Autodesk Inventor part; units mm, degrees
ref_plane "YZ Plane" through (0, 0, 0) normal (1, 0, 0) x (0, 1, 0)
ref_plane "XZ Plane" through (0, 0, 0) normal (0, 1, 0) x (-1, 0, 0)
ref_plane "XY Plane" through (0, 0, 0) normal (0, 0, 1) x (1, 0, 0)
sketch "Panel" plane through (0, 0, 0) normal (0, 0, 1) x (1, 0, 0)
  line L0 (-190.5, 127) -> (190.5, 127)
  line L1 (190.5, 127) -> (190.5, -127)
  line L2 (190.5, -127) -> (-190.5, -127)
  line L3 (-190.5, -127) -> (-190.5, 127)
  point P0 (0, 0)
  point P1 (-190.5, 0)
  point P2 (0, 127)
  dimension "d0" = 254
  dimension "d3" = 381
sketch "JoystickMount" plane through (0, 0, 0) normal (0, 0, 1) x (1, 0, 0)
  line L0 (-114.625, 55.25) -> (-114.625, 14.75) construction
  line L1 (-114.625, 14.75) -> (-29.625, 14.75) construction
  point P0 (0, 0)
  point P1 (-72.125, 35)
  point P2 (-29.625, 55.25)
  point P3 (-114.625, 35)
  point P4 (-72.125, 14.75)
  dimension "d4" = 40.5
  dimension "d6" = 85
  dimension "d19" = 35
  dimension "d45" = 72.125
sketch "ButtonMounts" plane through (0, 0, 0) normal (0, 0, 1) x (1, 0, 0)
  line L0 (54.125, 74) -> (54.125, 35) construction
  line L1 (54.125, 35) -> (90.125, 35) construction
  point P0 (0, 0)
  point P1 (22.875, 56)
  point P2 (22.875, 17)
  point P3 (90.125, 74)
  point P4 (125.125, 65)
  point P5 (125.125, 26)
  point P6 (-72.125, 35)
  point P7 (72.125, 54.5)
  point P8 (54.125, 54.5)
  point P9 (72.125, 35)
  dimension "d7" = 39
  dimension "d9" = 39
  dimension "d10" = 39
  dimension "d11" = 39
  dimension "d12" = 31.25
  dimension "d13" = 36
  dimension "d14" = 35
  dimension "d15" = 18
  dimension "d16" = 9
  dimension "d55" = 144.25
  dimension "d56" = 72.125
extrude "PanelExtrusion" add sketch "Panel" against normal blind 3.175
hole "JoystickScrews" at (-29.625, 14.75, 0) at (-29.625, 55.25, 0) at (-114.625, 55.25, 0) at (-114.625, 14.75, 0) direction (0, 0, -1) diameter 4.5 end through all countersink diameter 9.4 countersink angle 90
hole "JoystickShaft" at (-72.125, 35, 0) direction (0, 0, -1) diameter 24 end through all
hole "ButtonHoles" at (125.125, 26, 0) at (90.125, 35, 0) at (90.125, 74, 0) at (125.125, 65, 0) at (54.125, 74, 0) at (54.125, 35, 0) at (22.875, 56, 0) at (22.875, 17, 0) direction (0, 0, -1) diameter 30 end through all
fillet "Corners" radius 1 4 edges at (190.5, 127, -1.5875) (190.5, -127, -1.5875) (-190.5, 127, -1.5875) (-190.5, -127, -1.5875)
ref_plane "10DegOffsetAlignment" through (190.5, -127, -3.175) normal (0, -0.9848, 0.1736) x (-1, 0, 0)
sketch "ScrewHoleCenters" plane through (0, 0, 0) normal (0, 0, 1) x (1, 0, 0)
  line L0 (-190.5, -126) -> (-190.5, 126)
  line L1 (-177.8, 89.411) -> (-180.975, 89.411)
  line L2 (-180.975, 85.6137) -> (-177.8, 85.6137)
  line L3 (-177.8, -85.9663) -> (-180.975, -85.9663)
  line L4 (-180.975, -89.7636) -> (-177.8, -89.7636)
  line L5 (177.8, -89.7636) -> (180.975, -89.7636)
  line L6 (180.975, -85.9663) -> (177.8, -85.9663)
  line L7 (177.8, 85.6137) -> (180.975, 85.6137)
  line L8 (180.975, 89.411) -> (177.8, 89.411)
  line L9 (-180.975, 89.411) -> (-180.975, 85.6137) construction
  line L10 (-177.8, 85.6137) -> (-177.8, 89.411) construction
  line L11 (-180.975, -85.9663) -> (-180.975, -89.7636) construction
  line L12 (-177.8, -89.7636) -> (-177.8, -85.9663) construction
  line L13 (177.8, -89.7636) -> (177.8, -85.9663) construction
  line L14 (180.975, -85.9663) -> (180.975, -89.7636) construction
  line L15 (177.8, 85.6137) -> (177.8, 89.411) construction
  line L16 (180.975, 89.411) -> (180.975, 85.6137) construction
  point P0 (0, 0)
  point P1 (-179.3875, 87.5123)
  point P2 (-177.8, 87.5123)
  point P3 (-179.3875, 85.6137)
  point P4 (-179.3875, -87.865)
  point P5 (179.3875, -87.865)
  point P6 (179.3875, 87.5123)
  point P7 (-179.3875, -89.7636)
  point P8 (-180.975, -87.865)
  point P9 (177.8, -87.865)
  point P10 (179.3875, -89.7636)
  point P11 (179.3875, 85.6137)
  point P12 (177.8, 87.5123)
hole "PanelBoltHoles" at (-179.3875, 87.5123, 0) at (-179.3875, -87.865, 0) at (179.3875, -87.865, 0) at (179.3875, 87.5123, 0) direction (0, 0, -1) diameter 3.7973 end through all
sketch "TabSlotSketch" plane through (0, 0, 0) normal (0, 0, 1) x (1, 0, 0)
  circle A0 centre (179.3875, -87.865) radius 1.8986
  circle A1 centre (-179.3875, 87.5123) radius 1.8986
  circle A2 centre (-179.3875, -87.865) radius 1.8986
  circle A3 centre (179.3875, 87.5123) radius 1.8986
  line L0 (190.5, 126) -> (190.5, -126)
  line L1 (-190.5, -126) -> (-190.5, 126)
  line L2 (-179.3875, 87.5123) -> (-179.3875, -87.865) construction
  line L3 (179.3875, 87.5123) -> (179.3875, -87.865) construction
  line L4 (-181.229, 12.7777) -> (-177.546, 12.7777)
  line L5 (-177.546, 12.7777) -> (-177.546, -13.1303)
  line L6 (-177.546, -13.1303) -> (-181.229, -13.1303)
  line L7 (-181.229, -13.1303) -> (-181.229, 12.7777)
  line L8 (181.229, -13.1303) -> (177.546, -13.1303)
  line L9 (177.546, -13.1303) -> (177.546, 12.7777)
  line L10 (177.546, 12.7777) -> (181.229, 12.7777)
  line L11 (181.229, 12.7777) -> (181.229, -13.1303)
  point P0 (0, 0)
  point P1 (-179.3875, -0.1763)
  point P2 (-181.229, -0.1763)
  point P3 (-179.3875, -13.1303)
  point P4 (179.3875, -0.1763)
  point P5 (181.229, -0.1763)
  point P6 (179.3875, 12.7777)
  point P7 (-179.3875, -0.1763)
  point P8 (179.3875, -0.1763)
  dimension "d66" = 25.908
  dimension "d68" = 3.683
  dimension "d69" = 25.908
  dimension "d70" = 3.683
extrude "TabSlotExtrusion" cut sketch "TabSlotSketch" against normal blind 3.175 contours L4 L5 L6 L7 | L8 L9 L10 L11
fillet "TabSlotFillets" radius 0.5 8 edges at (-177.546, 12.7777, -1.5875) (-181.229, 12.7777, -1.5875) (-177.546, -13.1303, -1.5875) (-181.229, -13.1303, -1.5875) (181.229, 12.7777, -1.5875) (177.546, 12.7777, -1.5875) (177.546, -13.1303, -1.5875) (181.229, -13.1303, -1.5875)
equation "\"d59\" = ScrewHoleD"
equation "\"d66\" = SlotLength"
equation "\"d68\" = SlotWidth"
equation "\"d69\" = SlotLength"
equation "\"d70\" = SlotWidth"
equation "\"d73\" = SlotFilletRad"
properties part number "Panel_top_2" material "Aluminum"
Check sheet for the modelled part. Datum: model origin and axes. Units: mm. Give positions to 0.01 mm unless a question says otherwise; leave off trailing zeros. Order: outer loops, then holes, each group sorted by start corner. A loop starts at its lowest first (then second) coordinate and runs counter-clockwise, first axis right, second up. Notation, with made-up numbers: (-32.75, 18) - (15.25, 18) arc R19 ccw to (15.25, 40) - close; hole circle Ø2 at (-21.5, 70). An arc over 180 degrees is marked (long way). Answer as CSV lines item,"result".
1. Scan lines: probe 1 along X at (y, z) = (-12, -0.5); probe 2 along Y at (x, z) = (103, -3); probe 3 along X at (y, z) = (35, -1.65) (3 decimals). Record each from-to range of solid material in increasing order. Write a range as from..to.
Result sheet:
probe 1,"-190.5..-181.23, -177.55..177.55, 181.23..190.5"
probe 2,"-127..27.3, 42.7..66.3, 81.7..127"
probe 3,"-190.5..-84.125, -60.125..39.125, 69.125..75.125, 105.125..113.125, 137.125..190.5"
2. Section check B-B (z = -1.65). State how many separate pieces and enclosed holes the cut face has, then the cut area to 3 significant figures.
Result sheet:
separate pieces,"1"
enclosed holes,"19"
area,"90,300 mm²"
3. Mould release check, pull along X, two halves, no side actions. Record for faces 1 (the face through (-3, 2, 0)), 2 (the face through (22.215, 70.985, -1.61)): released by +X, released by -X, zero draft, split by the parting line, or undercut.
Result sheet:
face 1,"zero draft"
face 2,"undercut"
4. Go/stop test with flat-tipped pins: P1, Ø5, axis at x = -29.625, y = 14.75, coming from the +Z side; P2, Ø2, axis at x = -81, y = -55.5, coming from the +Z side; P3, Ø6, axis at x = -114.625, y = 55.25, coming from the +Z side. Record where each tip stops, or that it passes through.
Result sheet:
P1,"z = -2.2"
P2,"z = 0"
P3,"z = -1.7"
5. Section check A-A (y = 65). Record the boundary of the cut face in (x, z) (3 decimals).
Result sheet:
outline,"(-190.5, -3.175) - (10.875, -3.175) - (10.875, 0) - (-190.5, 0) - close; (34.875, -3.175) - (42.125, -3.175) - (42.125, 0) - (34.875, 0) - close; (66.125, -3.175) - (78.125, -3.175) - (78.125, 0) - (66.125, 0) - close; (102.125, -3.175) - (110.125, -3.175) - (110.125, 0) - (102.125, 0) - close; (140.125, -3.175) - (190.5, -3.175) - (190.5, 0) - (140.125, 0) - close"
